Could you check a few things on this drawing? It's one solid part, dimensions in mm from its lowest x, y, z. Round coordinates to 2 decimals unless told otherwise and drop trailing zeros. Loops run counter-clockwise (first coordinate to the right, second up) from the corner with the lowest first, then second, coordinate; pieces in that order, holes last. Notation, with made-up numbers: (54.5, -21.75) -> (95.5, -21.75) arc R23 cw to (95.5, 13.25) -> close; hole circle Ø7 at (13.5, -1.5). An arc over 180 degrees is marked (long way). Use one line per item in the form item = value. Start each with the question number.
Item 1: Thinking about a two-plate mould opening in Y: for the marked faces 1, 2 and 3, which applies, released by +Y, released by -Y, zero draft, split by the parting line, or undercut?
Item 2: If I drill on L1, parallel to Z at x = 23, y = 8; L2, parallel to Y at x = 10.75, z = 10; L3, parallel to Y at x = 5.5, z = 7, over which ranges is the centre line in solid material (lowest first)? Write a range as [from, to].
Item 3: I'm going to push a flat-ended pin straight in: pin 1 Ø10 at (x, z) = (23, 9.5) entering from -Y. Where does the tip first touch, or does it pass through?
Item 4: If we section it at B-B (z = 10): Write out the boundary of the cut face in (x, y), then the cut area to 3 significant figures.
Item 5: If we section it at A-A (y = 8): Write out the boundary of the cut face in (x, z).
Item 6: If we section it at C-C (x = 27.5): Write out the boundary of the cut face in (y, z).
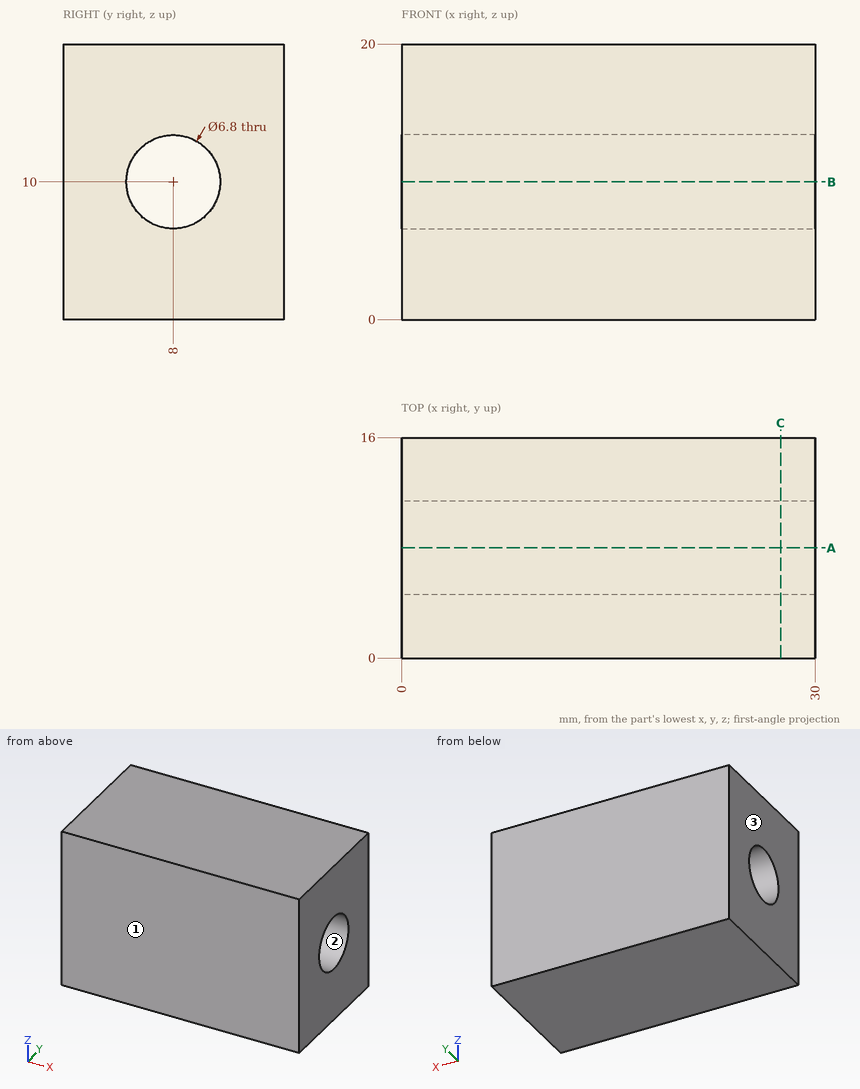
Values found:
q1.face_1 = released by -Y
q1.face_2 = undercut
q1.face_3 = zero draft
q2.L1 = [0, 6.6], [13.4, 20]
q2.L2 = [0, 4.6], [11.4, 16]
q2.L3 = [0, 6.4], [9.6, 16]
q3.pin_1 = 0
q4.outline = (0, 0) -> (30, 0) -> (30, 4.6) -> (0, 4.6) -> close; (0, 11.4) -> (30, 11.4) -> (30, 16) -> (0, 16) -> close
q4.area = 276 mm2
q5.outline = (0, 0) -> (30, 0) -> (30, 6.6) -> (0, 6.6) -> close; (0, 13.4) -> (30, 13.4) -> (30, 20) -> (0, 20) -> close
q6.outline = (0, 0) -> (16, 0) -> (16, 20) -> (0, 20) -> close; hole circle Ø6.8 at (8, 10)
